The model under review builds one solid part; all positions refer to its coordinate system, in mm. Face numbers are marked on the shaded views. Coordinates: 2 decimals unless noted, no trailing zeros. Write each loop counter-clockwise with the first axis right and the second up, starting at its lowest first coordinate (ties: lowest second). Pieces come first, ordered by that corner, then holes. Notation, with made-up numbers: M 86,88.5 L 125,88.5 A14 cw 125,92.5 Z; hole C -20.75,78.25 d11. An arc over 180 degrees is marked long. Answer as a JSON object with one key per item and string values.
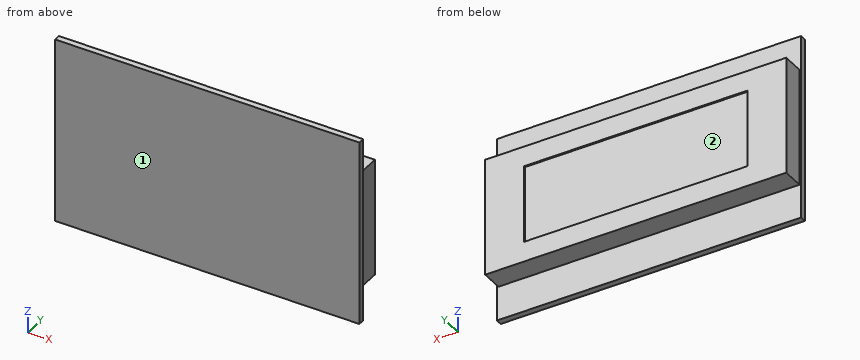
```python
from build123d import *

# Parameters (mm, degrees)
SKETCH1_W           = 98
SKETCH1_H           = 60
BOSS_EXTRUDE1_DEPTH = 2
SKETCH2_W           = 97
SKETCH2_H           = 38
BOSS_EXTRUDE2_DEPTH = 7
SKETCH4_W           = 72
SKETCH4_H           = 25
CUT_EXTRUDE1_DEPTH  = 0.5


with BuildPart() as part:
    # Sketch1 → Boss-Extrude1 (new body)
    with BuildSketch(Plane(origin=(0, 0, 0), x_dir=(1, 0, 0), z_dir=(0, 1, 0))):
        Rectangle(SKETCH1_W, SKETCH1_H)
    extrude(amount=BOSS_EXTRUDE1_DEPTH)

    # Sketch2 → Boss-Extrude2 (add)
    with BuildSketch(Plane(origin=(0, 2, 0), x_dir=(1, 0, 0), z_dir=(0, 1, 0))):
        Rectangle(SKETCH2_W, SKETCH2_H)
    extrude(amount=BOSS_EXTRUDE2_DEPTH)

    # Sketch4 → Cut-Extrude1 (cut)
    with BuildSketch(Plane(origin=(0, 9, 0), x_dir=(1, 0, 0), z_dir=(0, 1, 0))):
        Rectangle(SKETCH4_W, SKETCH4_H)
    extrude(amount=-CUT_EXTRUDE1_DEPTH, mode=Mode.SUBTRACT)


solid = part.part
```
(1) Draft analysis for pull direction X (two halves, no side actions). For the marked faces 1 and 2, state which applies: released by +X, released by -X, zero draft, split by the parting line, or undercut.
Results list:
{"face 1": "zero draft", "face 2": "undercut"}
(2) Add section B-B on x = 17.5. Give the boundary of the cut face in (y, z), and give its area (4 significant figures).
Results list:
{"outline": "M 0,-30 L 2,-30 L 2,-19 L 9,-19 L 9,-12.5 L 8.5,-12.5 L 8.5,12.5 L 9,12.5 L 9,19 L 2,19 L 2,30 L 0,30 Z", "area": "373.5 mm²"}
(3) For pin 1 Ø8 at (x, z) = (-8, 5) entering from +Y; pin 2 Ø3.5 at (y, z) = (5.5, 8.5) entering from -X; pin 3 Ø2 at (y, z) = (5.5, -20.5) entering from -X; pin 4 Ø2 at (y, z) = (5.5, -6.5) entering from +X, all flat-tipped, find the tip position at first contact; note any pin that passes through.
Results list:
{"pin 1": "y = 8.5", "pin 2": "x = -48.5", "pin 3": "through", "pin 4": "x = 48.5"}
(4) Wall thickness on line 1 along Z through (x, y) = (-27, 4.75); line 2 along X through (y, z) = (3.5, -16); line 3 along Y through (x, z) = (27, 25.5): over which ranges is each line inside the solid? List them lowest first. Write a range as from..to.
Results list:
{"line 1": "-19..19", "line 2": "-48.5..48.5", "line 3": "0..2"}
(5) Add section D-D on z = -26. Give the boundary of the cut face in (x, y).
Results list:
{"outline": "M -49,0 L 49,0 L 49,2 L -49,2 Z"}
(6) Add section C-C on y = 7. Give the boundary of the cut face in (x, z).
Results list:
{"outline": "M -48.5,-19 L 48.5,-19 L 48.5,19 L -48.5,19 Z"}
(7) Add section A-A on z = 3. Give the boundary of the cut face in (x, y), and give its area (3 significant figures).
Results list:
{"outline": "M -49,0 L 49,0 L 49,2 L 48.5,2 L 48.5,9 L 36,9 L 36,8.5 L -36,8.5 L -36,9 L -48.5,9 L -48.5,2 L -49,2 Z", "area": "839 mm²"}
